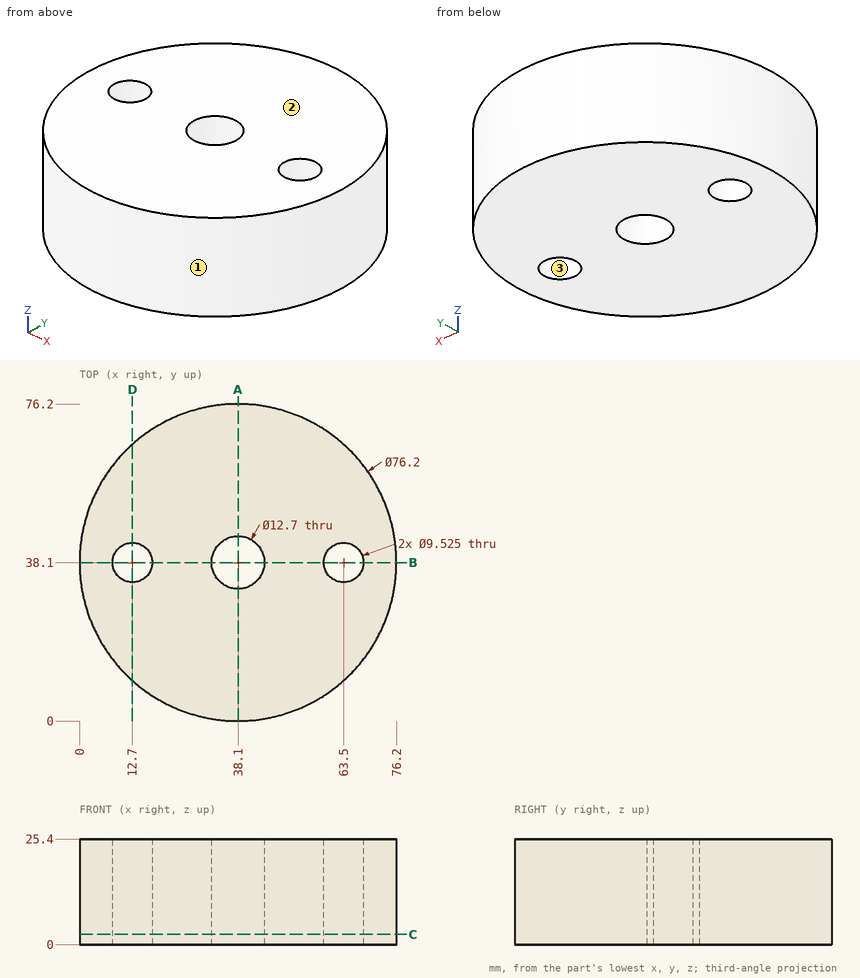
Could you check a few things on this drawing? It's one solid part, dimensions in mm from its lowest x, y, z. Round coordinates to 2 decimals unless told otherwise and drop trailing zeros. Write each loop counter-clockwise with the first axis right and the second up, starting at its lowest first coordinate (ties: lowest second). Pieces come first, ordered by that corner, then holes. Notation, with made-up numbers: (-21.5, 38.5) -> (14.5, 38.5) arc R21 ccw to (14.5, 62.5) -> close; hole circle Ø5 at (-11, 12.5). An arc over 180 degrees is marked (long way). Use a Markdown table: item, result.
1. We'd pull the mould along X, two halves only. Please class the marked faces 1, 2 and 3: +X half, -X half, draft (parallel to the pull), parting line (faces both ways), or undercut.
Answer key:
| item | result |
|---|---|
| face 1 | parting line |
| face 2 | draft |
| face 3 | undercut |
2. For pin 1 Ø2 at (x, z) = (54.5, 4.5) entering from -Y; pin 2 Ø10 at (y, z) = (23.5, 6.5) entering from +X; pin 3 Ø1 at (y, z) = (51, 22.5) entering from -X, each with a flat end and sliding along its axis, tell me the tip position at first contact or that it passes through.
Answer key:
| item | result |
|---|---|
| pin 1 | stops at y = 3.25 |
| pin 2 | stops at x = 74.97 |
| pin 3 | stops at x = 2.07 |
3. If we section it at D-D (x = 12.7): List the corners of the cut face in (y, z) for me, then the cut area to 3 significant figures.
Answer key:
| item | result |
|---|---|
| outline | (9.7, 0) -> (33.34, 0) -> (33.34, 25.4) -> (9.7, 25.4) -> close; (42.86, 0) -> (66.5, 0) -> (66.5, 25.4) -> (42.86, 25.4) -> close |
| area | 1,200 mm^2 |
4. If we section it at B-B (y = 38.1): List the corners of the cut face in (x, z) for me.
Answer key:
| item | result |
|---|---|
| outline | (0, 0) -> (7.94, 0) -> (7.94, 25.4) -> (0, 25.4) -> close; (17.46, 0) -> (31.75, 0) -> (31.75, 25.4) -> (17.46, 25.4) -> close; (44.45, 0) -> (58.74, 0) -> (58.74, 25.4) -> (44.45, 25.4) -> close; (68.26, 0) -> (76.2, 0) -> (76.2, 25.4) -> (68.26, 25.4) -> close |
5. If we section it at A-A (x = 38.1): List the corners of the cut face in (y, z) for me.
Answer key:
| item | result |
|---|---|
| outline | (0, 0) -> (31.75, 0) -> (31.75, 25.4) -> (0, 25.4) -> close; (44.45, 0) -> (76.2, 0) -> (76.2, 25.4) -> (44.45, 25.4) -> close |
6. Please list where these lines run through material, in increasing order: probe 1 along X at (y, z) = (38, 10.5); probe 2 along X at (y, z) = (38.5, 14); probe 3 along Y at (x, z) = (38.1, 5.5).
Answer key:
| item | result |
|---|---|
| probe 1 | x = 0 to 7.94, 17.46 to 31.75, 44.45 to 58.74, 68.26 to 76.2 |
| probe 2 | x = 0 to 7.95, 17.45 to 31.76, 44.44 to 58.75, 68.25 to 76.2 |
| probe 3 | y = 0 to 31.75, 44.45 to 76.2 |
7. If we section it at C-C (z = 2.5): State how many separate pieces and enclosed holes the cut face has, then the cut area to 3 significant figures.
Answer key:
| item | result |
|---|---|
| separate pieces | 1 |
| enclosed holes | 3 |
| area | 4,290 mm^2 |
